Autodesk Inventor part; units mm, degrees
ref_plane "Work Plane1" through (0, 0, -3) normal (0, 0, 1) x (1, 0, 0)
ref_plane "YZ Plane" through (0, 0, 0) normal (1, 0, 0) x (0, 1, 0)
ref_plane "XZ Plane" through (0, 0, 0) normal (0, 1, 0) x (-1, 0, 0)
ref_plane "Work Plane1" through (0, 0, -3) normal (0, 0, 1) x (1, 0, 0)
sketch "Sketch1" plane through (0, 0, -3) normal (0, 0, 1) x (1, 0, 0)
  circle A0 centre (0, 0) radius 2.75
extrude "Extrusion3" add sketch "Sketch1" along normal blind 3
fillet "Fillet1" radius 0.1 2 edges at (-2.75, 0, -3) (-2.75, 0, 0)
sketch "Sketch2" plane through (0, 0, -3) normal (0, 0, 1) x (1, 0, 0)
  line L0 (-0.7217, 1.25) -> (0.7217, 1.25)
  line L1 (0.7217, -1.25) -> (-0.7217, -1.25)
  line L2 (-0.7217, -1.25) -> (-1.4434, 0)
  line L3 (0.7217, 1.25) -> (1.4434, 0)
  line L4 (-1.4434, 0) -> (-0.7217, 1.25)
  line L5 (1.4434, 0) -> (0.7217, -1.25)
extrude "Extrusion2" cut sketch "Sketch2" along normal blind 3
sketch "Sketch3" plane through (0, 0, 0) normal (0, 0, 1) x (1, 0, 0)
  circle A0 centre (0, 0) radius 1.5
extrude "Extrusion1" add sketch "Sketch3" along normal blind 8
chamfer "Chamfer1" distance 0.2 angle 45 1 edges at (-1.5, 0, 8)
thread "Thread1"
properties part number "DIN 912 M3 8 mm" material "Stainless Steel"
Verification items for the finished model (mm, model axes). A direction names the side the tool comes from. Coordinates: 2 decimals unless noted, no trailing zeros. Order: outer loops, then holes, each group sorted by start corner. A loop starts at its lowest first (then second) coordinate and runs counter-clockwise, first axis right, second up. Notation, with made-up numbers: (74.5, -13.5) -> (132.5, -13.5) arc R16 cw to (132.5, -4.5) -> close; hole circle Ø7 at (62.5, 1). An arc over 180 degrees is marked (long way). Put each result on its own line as item: value. Start each with the question number.
1. Mould release check, pull along Y, two halves, no side actions. Record for faces 4 (the flat face through (0, 1.25, -2)), 5 (the flat face through (0, 0, 8)), 6 (the cylindrical face through (-0.596, 2.685, -1.52)), 7 (the flat face through (-1.088, 0.616, -1.521)): released by +Y, released by -Y, zero draft, split by the parting line, or undercut.
2. Cross-section at C-C, the plane z = 5.25. Record the boundary of the cut face in (x, y).
3. Cross-section at A-A, the plane z = -1.5. Record the boundary of the cut face in (x, y), then the cut area to 3 significant figures.
4. Cross-section at B-B, the plane x = 0. Record the boundary of the cut face in (y, z), then the cut area to 3 significant figures.
5. Material ranges on L1, parallel to Z at x = 0.55, y = 0.1; L2, parallel to Z at x = 2.1, y = 1.2; L3, parallel to X at y = -0.9, z = -0.25, recorded low to high. Write a range as [from, to].
6. Access from +Z, -Z, +X, -X, +Y, -Y to the whole of each face (thin tool, end or side, straight path). Record for faces 1 (the flat face through (1.1, -1.1, -3)), 2 (the flat face through (1.08, 0.63, -1.52)), 3 (the cylindrical face through (-1.5, -0.07, 3.85)).
7. Go/stop test with flat-tipped pins: pin 1 Ø2 at (y, z) = (0, 2) entering from +X; pin 2 Ø0.8 at (x, y) = (0.5, 0.5) entering from -Z. Record where each tip stops, or that it passes through.
Computed:
1. face 4: undercut
1. face 5: zero draft
1. face 6: split by the parting line
1. face 7: undercut
2. outline: circle Ø3 at (0, 0)
3. outline: circle Ø5.5 at (0, 0); hole (-1.44, 0) -> (-0.72, -1.25) -> (0.72, -1.25) -> (1.44, 0) -> (0.72, 1.25) -> (-0.72, 1.25) -> close
3. area: 18.3 mm2
4. outline: (-2.75, -2.9) arc R0.1 ccw to (-2.65, -3) -> (-1.25, -3) -> (-1.25, 0) -> (1.25, 0) -> (1.25, -3) -> (2.65, -3) arc R0.1 ccw to (2.75, -2.9) -> (2.75, -0.1) arc R0.1 ccw to (2.65, 0) -> (1.5, 0) -> (1.5, 7.8) -> (1.3, 8) -> (-1.3, 8) -> (-1.5, 7.8) -> (-1.5, 0) -> (-2.65, 0) arc R0.1 ccw to (-2.75, -0.1) -> close
4. area: 33.0 mm2
5. L1: [0, 8]
5. L2: [-3, 0]
5. L3: [-2.6, -0.92], [0.92, 2.6]
6. face 1: -Z, +X, -X, +Y, -Y
6. face 2: -Z
6. face 3: +Z
7. pin 1: x = 1.5
7. pin 2: z = 0
